```python
from build123d import *

# Parameters (mm, degrees)
BOSS_EXTRUDE1_DEPTH = 15
SCALE1_SCALE        = 0.6


with BuildPart() as part:
    # Sketch1 → Boss-Extrude1 (new body)
    with BuildSketch(Plane(origin=(0, 0, 0), x_dir=(1, 0, 0), z_dir=(0, 1, 0))):
        Polygon((0, 358.35), (0, 7.5), (20.180404561, 7.5), (20.180404561, -7.5), (0, -7.5), (0, -358.35), (35.650600343, -358.35), (54.572500068, -34.997934227), (31.19655837, 0), (54.572500068, 34.997934227), (35.650600343, 358.35), align=None)
    extrude(amount=BOSS_EXTRUDE1_DEPTH)


with BuildPart() as part_1:
    # Scale1: scaled about (22.921989844, 7.5, 0)
    add(part.part.scale(SCALE1_SCALE).moved(Location((9.168795938, 3, 0))))


solid = part_1.part
```
CAD build for the part. Positions are in the model's coordinates, mm. A direction names the side the tool comes from. Round coordinates to 2 decimals unless told otherwise and drop trailing zeros. Order: outer loops, then holes, each group sorted by start corner. A loop starts at its lowest first (then second) coordinate and runs counter-clockwise, first axis right, second up.
Item 1: Pin check, flat tips, straight feed: pin 1 (5 mm diameter, centred on y = 8, z = -11.5, fed in from +X); pin 2 (4 mm diameter, centred on y = 10, z = -47.5, fed in from +X). Stop position of each tip, or through.
Item 2: Probe line 1 along Z through (x, y) = (19.5, 8.25); line 2 along Z through (x, y) = (28.5, 7); line 3 along X through (y, z) = (6.5, -130.5). List the from-to ranges inside material, lowest first.
Item 3: Saw through at D-D on z = -59. Write the cut outline in (x, y), then the cut area to 3 significant figures.
Item 4: Tool access for faces 1 (the face through (35, 7.44, 10.65)), 2 (the face through (20, 7, -215.01)), 3 (the face through (15, 7, 4.5)): list every direction of +Z, -Z, +X, -X, +Y, -Y with a clear straight run to the whole face (end or side of a thin tool).
Item 5: Saw through at B-B on y = 5.5. Write the cut outline in (x, z), then the cut area to 3 significant figures.
Item 6: Saw through at C-C on x = 36.5. Write the cut outline in (y, z), then the cut area to 3 significant figures.
Item 7: Saw through at A-A on x = 15. Write the cut outline in (y, z), then the cut area to 3 significant figures.
Reported:
1. pin 1: stops at x = 37.24
1. pin 2: stops at x = 40.48
2. line 1: z = -215.01 to -4.5, 4.5 to 215.01
2. line 2: z = -215.01 to -0.92, 0.92 to 215.01
2. line 3: x = 9.17 to 35.5
3. outline: (9.17, 3) - (39.69, 3) - (39.69, 12) - (9.17, 12) - close
3. area: 275 mm2
4. face 1: +X, +Y, -Y
4. face 2: -Z, +X, -X, +Y, -Y
4. face 3: -X, +Y, -Y
5. outline: (9.17, -215.01) - (30.56, -215.01) - (41.91, -21) - (27.89, 0) - (41.91, 21) - (30.56, 215.01) - (9.17, 215.01) - (9.17, 4.5) - (21.28, 4.5) - (21.28, -4.5) - (9.17, -4.5) - close
5. area: 11,500 mm2
6. outline: (3, -113.49) - (12, -113.49) - (12, -12.9) - (3, -12.9) - close; (3, 12.9) - (12, 12.9) - (12, 113.49) - (3, 113.49) - close
6. area: 1,810 mm2
7. outline: (3, -215.01) - (12, -215.01) - (12, -4.5) - (3, -4.5) - close; (3, 4.5) - (12, 4.5) - (12, 215.01) - (3, 215.01) - close
7. area: 3,790 mm2
